Here's how the part is built. I have some questions about the finished solid (model axes, mm). A direction names the side the tool comes from. Round coordinates to 2 decimals unless told otherwise and drop trailing zeros. Order: outer loops, then holes, each group sorted by start corner. A loop starts at its lowest first (then second) coordinate and runs counter-clockwise, first axis right, second up.
```python
from build123d import *

# Parameters (mm, degrees)
SKETCH1_W                   = 45
SKETCH1_H                   = 14.46
BOSS_EXTRUDE1_DEPTH         = 3
F_1_4_0_25_DIAMETER_HOLE1_D = 6.35
SKETCH5_W                   = 24.2
SKETCH5_H                   = 37.04
BOSS_EXTRUDE2_DEPTH         = 3
SKETCH6_W                   = 15.5
SKETCH6_H                   = 30
BOSS_EXTRUDE3_DEPTH         = 5
BOSS_EXTRUDE4_START         = -29.2
SKETCH7_W                   = 15.5
SKETCH7_H                   = 30
BOSS_EXTRUDE4_DEPTH         = 5
SKETCH12_W                  = 24.2
SKETCH12_H                  = 20.5
CUT_EXTRUDE1_DEPTH          = 3
M5_CLEARANCE_HOLE1_D        = 5.5
FILLET3_R                   = 2.5
FILLET4_R                   = 2.5


with BuildPart() as part:
    # Sketch1 → Boss-Extrude1 (new body)
    with BuildSketch(Plane.XY):
        with Locations((13.988651535, -1.802042724)):
            Rectangle(SKETCH1_W, SKETCH1_H)
    extrude(amount=BOSS_EXTRUDE1_DEPTH)

    # 1/4 (0.25) Diameter Hole1 (through all)
    with Locations(Plane(origin=(0, 0, 0), x_dir=(-1, 0, 0), z_dir=(0, 0, -1))):
        with Locations((-26.488651535, -1.532042724), (-1.488651535, -1.532042724)):
            Hole(F_1_4_0_25_DIAMETER_HOLE1_D / 2)

    # Sketch5 → Boss-Extrude2 (add)
    with BuildSketch(Plane(origin=(0, 0, 0), x_dir=(-1, 0, 0), z_dir=(0, 0, -1))):
        with Locations((-13.988651535, 23.947957276)):
            Rectangle(SKETCH5_W, SKETCH5_H)
    extrude(amount=-BOSS_EXTRUDE2_DEPTH)

    # Sketch6 → Boss-Extrude3 (add)
    with BuildSketch(Plane.ZY.offset(-1.888651535)):
        with Locations((-4.75, 27.467957276)):
            Rectangle(SKETCH6_W, SKETCH6_H)
    extrude(amount=BOSS_EXTRUDE3_DEPTH)

    # Sketch7 → Boss-Extrude4 (add)
    with BuildSketch(Plane.ZY.offset(3.111348465).offset(BOSS_EXTRUDE4_START)):
        with Locations((-4.75, 27.467957276)):
            Rectangle(SKETCH7_W, SKETCH7_H)
    extrude(amount=-BOSS_EXTRUDE4_DEPTH)

    # Sketch12 → Cut-Extrude1 (cut)
    with BuildSketch(Plane(origin=(0, 0, 0), x_dir=(-1, 0, 0), z_dir=(0, 0, -1))):
        with Locations((-13.988651535, 32.217957276)):
            Rectangle(SKETCH12_W, SKETCH12_H)
    extrude(amount=-CUT_EXTRUDE1_DEPTH, mode=Mode.SUBTRACT)

    # M5 Clearance Hole1 (through all)
    with Locations(Plane.ZY.offset(3.111348465)):
        with Locations((-6.85, 37.467957276), (-6.85, 27.467957276)):
            Hole(M5_CLEARANCE_HOLE1_D / 2)

    # Fillet3
    fillet3_edges = [part.edges().sort_by_distance(p)[0] for p in [
        (-8.511348465, 5.427957276, 1.5),
        (36.488651535, 5.427957276, 1.5),
        (36.488651535, -9.032042724, 1.5),
        (-8.511348465, -9.032042724, 1.5),
    ]]
    fillet(fillet3_edges, radius=FILLET3_R)

    # Fillet4
    fillet4_edges = [part.edges().sort_by_distance(p)[0] for p in [
        (1.888651535, 5.427957276, 1.5),
        (26.088651535, 5.427957276, 1.5),
        (26.088651535, 12.467957276, 1.5),
        (1.888651535, 12.467957276, 1.5),
        (31.088651535, 12.467957276, -4.75),
        (-3.111348465, 12.467957276, -4.75),
        (28.588651535, 12.467957276, -12.5),
        (-0.611348465, 12.467957276, -12.5),
    ]]
    fillet(fillet4_edges, radius=FILLET4_R - 0.0001)  # a hair under: the kernel refuses the full size


solid = part.part
```
1. On a 3-axis mill with a long thin cutter (end or side, diameter ignored), from which of +Z, -Z, +X, -X, +Y, -Y can I reach the whole of each face in a straight line? I mean faces 1 (the cylindrical face through (1.137, 6.141, 1.521)), 2 (the flat face through (14, 21.968, 1)), 3 (the flat face through (26.089, 28, -3)). Say none if no direction works.
Evaluation:
face 1: +Z, -Z, -X
face 2: +Z, -Z, +Y
face 3: -Z, +Y
2. I need wall thicknesses on probe 1 along Y at (x, z) = (-0.6, -6.85); probe 2 along X at (y, z) = (32, -11); probe 3 along Y at (x, z) = (27.5, -8.25). Which ranges of each line are inside material? Lowest first, please.
Evaluation:
probe 1: y = 12.47 to 24.72, 30.22 to 34.72, 40.22 to 42.47
probe 2: x = -3.11 to 1.89, 26.09 to 31.09
probe 3: y = 12.47 to 25.1, 29.83 to 35.1, 39.83 to 42.47
3. If we mould it in two halves opening along Y, with no side actions, what happens to faces 4 (the cylindrical face through (29.517, -0.578, 1.521)), 5 (the flat face through (-1, 42.468, -5)), 6 (the cylindrical face through (35.776, -8.28, 1.521))? For each: released by +Y, released by -Y, zero draft, split by the parting line, or undercut.
Evaluation:
face 4: undercut
face 5: released by +Y
face 6: released by -Y
4. If we section it at B-B, the plane z = 1.25: State how many separate pieces and enclosed holes the cut face has, and give its area (3 significant figures).
Evaluation:
separate pieces: 1
enclosed holes: 2
area: 1,280 mm2
5. If we section it at C-C, the plane x = -5: Write out the boundary of the cut face in (y, z), and give its area (3 significant figures).
Evaluation:
outline: (-9.03, 0) - (5.43, 0) - (5.43, 3) - (-9.03, 3) - close
area: 43.4 mm2
6. If we section it at A-A, the plane z = -6.85: Write out the boundary of the cut face in (x, y), and give its area (3 significant figures).
Evaluation:
outline: (-3.11, 14.97) arc R2.5 ccw to (-0.61, 12.47) - (1.89, 12.47) - (1.89, 24.72) - (-3.11, 24.72) - close; (-3.11, 30.22) - (1.89, 30.22) - (1.89, 34.72) - (-3.11, 34.72) - close; (-3.11, 40.22) - (1.89, 40.22) - (1.89, 42.47) - (-3.11, 42.47) - close; (26.09, 12.47) - (28.59, 12.47) arc R2.5 ccw to (31.09, 14.97) - (31.09, 24.72) - (26.09, 24.72) - close; (26.09, 30.22) - (31.09, 30.22) - (31.09, 34.72) - (26.09, 34.72) - close; (26.09, 40.22) - (31.09, 40.22) - (31.09, 42.47) - (26.09, 42.47) - close
area: 187 mm2
7. I'm going to push flat-ended pins straight in: P1, Ø1, axis at y = 31, z = -1.5, coming from the +X side; P2, Ø9, axis at y = 37.47, z = -6.85, coming from the -X side; P3, Ø9.5, axis at x = 18.5, y = 0.5, coming from the -Z side. Where does each tip first touch, or does it pass through?
Evaluation:
P1: stops at x = 31.09
P2: stops at x = -3.11
P3: stops at z = 0
8. If we section it at D-D, the plane y = 11: Write out the boundary of the cut face in (x, z), and give its area (3 significant figures).
Evaluation:
outline: (1.67, 0) - (26.31, 0) - (26.31, 3) - (1.67, 3) - close
area: 73.9 mm2
